The model under review builds one solid part; all positions refer to its coordinate system, in mm. A direction names the side the tool comes from. Round coordinates to 2 decimals unless told otherwise and drop trailing zeros. Order: outer loops, then holes, each group sorted by start corner. A loop starts at its lowest first (then second) coordinate and runs counter-clockwise, first axis right, second up. Notation, with made-up numbers: M 66,73 L 114,73 A8 ccw 114,79 Z; hole C 20,13.25 d9. An arc over 180 degrees is marked long. Answer as a JSON object with one key per item and string values. Group by question number.
1) Consider section D-D, the plane x = -1.75. Write out the cut boundary in (y, z).
2) For faces 5 (the flat face through (-2, 0.5, -1)), 6 (the flat face through (2, 2.5, -1)), 7 (the flat face through (2, 3, -2)), list the 3-axis set-ups (+Z, -Z, +X, -X, +Y, -Y) from which the entire face can be reached by the end or side of a thin tool; tool diameter is ignored.
3) To check wall thickness, follow line 1 (X direction, y = 0.3, z = 0); line 2 (X direction, y = 2.75, z = -1.2); line 3 (X direction, y = 1.9, z = 0). State the ranges of each line that lie inside material, in increasing order.
4) Consider section C-C, the plane y = 1.45. Write out the cut boundary in (x, z).
5) Consider section B-B, the plane x = 0. Write out the cut boundary in (y, z).
6) Consider section A-A, the plane z = 0. Write out the cut boundary in (x, y), then the cut area to 3 significant figures.
7) The part is to be moulded in two halves that separate along X. For faces 1 (the cylindrical face through (0.9, 1.48, 2.86)), 2 (the cylindrical face through (2.44, 0.25, -0.54)), 3 (the flat face through (2, 0, -2)), 4 (the cylindrical face through (-1.952, 2.754, -0.434)), say which applies: +X half, -X half, draft (parallel to the pull), parting line (faces both ways), or undercut.
8) Insertion check: pin 1 Ø1.8 at (x, z) = (0, 0) entering from -Y. The pin has a flat end and moves straight along its axis. Give the tip position at first contact, or say it passes through.
```python
from build123d import *

# Parameters (mm, degrees)
SKETCH1_R           = 3
SKETCH1_R_2         = 1.5
BOSS_EXTRUDE1_DEPTH = 3
SKETCH2_R           = 2.5
SKETCH2_R_2         = 2
CUT_EXTRUDE1_DEPTH  = 0.5
CUT_EXTRUDE2_START  = -0.5
SKETCH3_R           = 2.5
SKETCH3_R_2         = 2
CUT_EXTRUDE2_DEPTH  = 0.5


with BuildPart() as part:
    # Sketch1 → Boss-Extrude1 (new body)
    with BuildSketch(Plane(origin=(0, 0, 0), x_dir=(1, 0, 0), z_dir=(0, 1, 0))):
        with Locations(Location((0, 0, 0), (0, 0, 270))):
            Circle(SKETCH1_R)
        with Locations(Location((0, 0, 0), (0, 0, 270))):
            Circle(SKETCH1_R_2, mode=Mode.SUBTRACT)
    extrude(amount=BOSS_EXTRUDE1_DEPTH)

    # Sketch2 → Cut-Extrude1 (cut)
    with BuildSketch(Plane(origin=(0, 3, 0), x_dir=(1, 0, 0), z_dir=(0, 1, 0))):
        with Locations(Location((0, 0, 0), (0, 0, 270))):
            Circle(SKETCH2_R)
        with Locations(Location((0, 0, 0), (0, 0, 270))):
            Circle(SKETCH2_R_2, mode=Mode.SUBTRACT)
    extrude(amount=-CUT_EXTRUDE1_DEPTH, mode=Mode.SUBTRACT)

    # Sketch3 → Cut-Extrude2 (cut)
    with BuildSketch(Plane(origin=(0, 0, 0), x_dir=(-1, 0, 0), z_dir=(0, -1, 0)).offset(CUT_EXTRUDE2_START)):
        with Locations(Location((0, 0, 0), (0, 0, 270))):
            Circle(SKETCH3_R)
        with Locations(Location((0, 0, 0), (0, 0, 270))):
            Circle(SKETCH3_R_2, mode=Mode.SUBTRACT)
    extrude(amount=CUT_EXTRUDE2_DEPTH, mode=Mode.SUBTRACT)


solid = part.part
```
Results list:
{
 "1": {"outline": "M 0,-2.44 L 3,-2.44 L 3,-1.79 L 2.5,-1.79 L 2.5,-0.97 L 3,-0.97 L 3,0.97 L 2.5,0.97 L 2.5,1.79 L 3,1.79 L 3,2.44 L 0,2.44 L 0,1.79 L 0.5,1.79 L 0.5,0.97 L 0,0.97 L 0,-0.97 L 0.5,-0.97 L 0.5,-1.79 L 0,-1.79 Z"},
 "2": {"face 5": "-Y", "face 6": "+Y", "face 7": "+Z, -Z, +X, -X, +Y"},
 "3": {"line 1": "-3 to -2.5, -2 to -1.5, 1.5 to 2, 2.5 to 3", "line 2": "-2.75 to -2.19, -1.6 to -0.9, 0.9 to 1.6, 2.19 to 2.75", "line 3": "-3 to -1.5, 1.5 to 3"},
 "4": {"outline": "C 0,0 d6; hole C 0,0 d3"},
 "5": {"outline": "M 0,-3 L 3,-3 L 3,-2.5 L 2.5,-2.5 L 2.5,-2 L 3,-2 L 3,-1.5 L 0,-1.5 L 0,-2 L 0.5,-2 L 0.5,-2.5 L 0,-2.5 Z; M 0,1.5 L 3,1.5 L 3,2 L 2.5,2 L 2.5,2.5 L 3,2.5 L 3,3 L 0,3 L 0,2.5 L 0.5,2.5 L 0.5,2 L 0,2 Z"},
 "6": {"outline": "M -3,0 L -2.5,0 L -2.5,0.5 L -2,0.5 L -2,0 L -1.5,0 L -1.5,3 L -2,3 L -2,2.5 L -2.5,2.5 L -2.5,3 L -3,3 Z; M 1.5,0 L 2,0 L 2,0.5 L 2.5,0.5 L 2.5,0 L 3,0 L 3,3 L 2.5,3 L 2.5,2.5 L 2,2.5 L 2,3 L 1.5,3 Z", "area": "8.00 mm^2"},
 "7": {"face 1": "parting line", "face 2": "undercut", "face 3": "draft", "face 4": "undercut"},
 "8": {"pin 1": "through"}
}
